Verification items for the finished model (mm, model axes). A direction names the side the tool comes from. Give positions to 0.01 mm unless a question says otherwise; leave off trailing zeros. Loops run counter-clockwise (first coordinate to the right, second up) from the corner with the lowest first, then second, coordinate; pieces in that order, holes last. Notation, with made-up numbers: M 63.5,-39 L 99.5,-39 A15 cw 99.5,-24 Z; hole C 45.25,62.5 d5. An arc over 180 degrees is marked long. Answer in a Markdown table with one row per item.
```python
from build123d import *

# Parameters (mm, degrees)
F0_W      = 15
F0_H      = 14.771302
F1_DEPTH  = 15
F2_R      = 4.5
F3_DEPTH  = 13.75
F4_R      = 4.5
F5_DEPTH  = 13.75
F6_R      = 4.5
F7_DEPTH  = 13.75
F8_R      = 1.575
F9_DEPTH  = 15.001
F10_R     = 1.575
F11_DEPTH = 14.772302
F12_R     = 1.575
F13_DEPTH = 15.001


with BuildPart() as f1:
    # F0 (on Front) → F1 (new body)
    with BuildSketch(Plane.XZ):
        Rectangle(F0_W, F0_H)
    extrude(amount=F1_DEPTH)

    # F2 (on face) → F3 (cut)
    with BuildSketch(Plane.XZ.offset(15)):
        Circle(F2_R)
    extrude(amount=-F3_DEPTH, mode=Mode.SUBTRACT)

    # F4 (on face) → F5 (cut)
    with BuildSketch(Plane.XY.offset(7.385651)):
        with Locations((0, -7.5)):
            Circle(F4_R)
    extrude(amount=-F5_DEPTH, mode=Mode.SUBTRACT)

    # F6 (on face) → F7 (cut)
    with BuildSketch(Plane(origin=(-7.5, 0, 0), x_dir=(0, -1, 0), z_dir=(-1, 0, 0))):
        with Locations((7.5, 0)):
            Circle(F6_R)
    extrude(amount=-F7_DEPTH, mode=Mode.SUBTRACT)

    # F8 (on face) → F9 (cut, through all)
    with BuildSketch(Plane(origin=(0, 0, 0), x_dir=(-1, 0, 0), z_dir=(0, 1, 0))):
        Circle(F8_R)
    extrude(amount=-F9_DEPTH, mode=Mode.SUBTRACT)

    # F10 (on face) → F11 (cut, through all)
    with BuildSketch(Plane(origin=(0, 0, -7.385651), x_dir=(1, 0, 0), z_dir=(0, 0, -1))):
        with Locations((0, 7.5)):
            Circle(F10_R)
    extrude(amount=-F11_DEPTH, mode=Mode.SUBTRACT)

    # F12 (on face) → F13 (cut, through all)
    with BuildSketch(Plane.YZ.offset(7.5)):
        with Locations((-7.5, 0)):
            Circle(F12_R)
    extrude(amount=-F13_DEPTH, mode=Mode.SUBTRACT)


solid = f1.part
```
Item 1: Sectioned sample at A-A (y = -7.5). Record the cut outline in (x, z) (3 decimals), and give its area (3 significant figures).
Reported:
| item | result |
|---|---|
| outline | M -7.5,-7.386 L -1.575,-7.386 L -1.575,-6.364 L -4.5,-6.364 L -4.5,-4.5 L -7.5,-4.5 Z; M -7.5,4.5 L -4.5,4.5 L -4.5,7.386 L -7.5,7.386 Z; M 1.575,-7.386 L 7.5,-7.386 L 7.5,-1.575 L 6.25,-1.575 L 6.25,-4.5 L 4.5,-4.5 L 4.5,-6.364 L 1.575,-6.364 Z; M 4.5,4.5 L 6.25,4.5 L 6.25,1.575 L 7.5,1.575 L 7.5,7.386 L 4.5,7.386 Z |
| area | 47.9 mm^2 |
Item 2: Go/stop test with a flat-tipped pin: pin 1 (5.5 mm diameter, centred on x = 0, y = -7.5, fed in from +Z). Record where the tip stops, or that it passes through.
Reported:
| item | result |
|---|---|
| pin 1 | stops at z = -6.36 |
Item 3: Sectioned sample at C-C (x = 4). Record the cut outline in (y, z).
Reported:
| item | result |
|---|---|
| outline | M -15,-7.39 L 0,-7.39 L 0,7.39 L -5.44,7.39 L -5.44,4 A4.5 cw -3.5,2.06 L -1.25,2.06 L -1.25,-2.06 L -3.5,-2.06 A4.5 cw -5.44,-4 L -5.44,-6.36 L -9.56,-6.36 L -9.56,-4 A4.5 cw -11.5,-2.06 L -15,-2.06 Z; M -15,2.06 L -11.5,2.06 A4.5 cw -9.56,4 L -9.56,7.39 L -15,7.39 Z |
Item 4: Tool access check on faces 4 (the cylindrical face through (-0.59, -3.04, 5.78)), 5 (the cylindrical face through (-3.32, -13.35, 3.04)), 6 (the cylindrical face through (5.04, -4.18, 3.04)). Record the directions out of +Z, -Z, +X, -X, +Y, -Y that give a thin tool (end or side, any length) a straight path to the whole face; none if there is none.
Reported:
| item | result |
|---|---|
| face 4 | +Z |
| face 5 | -Y |
| face 6 | -X |
Item 5: Scan lines: L1, parallel to Y at x = 5.5, z = 0; L2, parallel to Z at x = 6.8, y = -7.5 (3 decimals); L3, parallel to Y at x = 0, z = -7.2 (3 decimals). Record each from-to range of solid material in increasing order. Write a range as [from, to].
Reported:
| item | result |
|---|---|
| L1 | y = [-15, -12], [-3, 0] |
| L2 | z = [-7.386, -1.575], [1.575, 7.386] |
| L3 | y = [-15, -9.075], [-5.925, 0] |
Item 6: Sectioned sample at D-D (z = 5.5). Record the cut outline in (x, y), and give its area (3 significant figures).
Reported:
| item | result |
|---|---|
| outline | M -7.5,-15 L 7.5,-15 L 7.5,0 L -7.5,0 Z; hole C 0,-7.5 d9 |
| area | 161 mm^2 |
Item 7: Release check for a two-part mould opening along Z. For faces 1 (the flat face through (-2, -7, -7.386)), 2 (the flat face through (-3.4, -10.7, 7.386)), 3 (the cylindrical face through (-3.32, -2.46, 3.04)) record: released by +Z, released by -Z, zero draft, split by the parting line, or undercut.
Reported:
| item | result |
|---|---|
| face 1 | released by -Z |
| face 2 | released by +Z |
| face 3 | undercut |
Item 8: Sectioned sample at B-B (z = 0). Record the cut outline in (x, y) (3 decimals).
Reported:
| item | result |
|---|---|
| outline | M -7.5,-15 L -4.5,-15 L -4.5,-12 L -7.5,-12 Z; M -7.5,-3 L -4.5,-3 L -4.5,-1.25 L -1.575,-1.25 L -1.575,0 L -7.5,0 Z; M 1.575,-1.25 L 4.5,-1.25 L 4.5,-3 L 6.25,-3 L 6.25,-5.925 L 7.5,-5.925 L 7.5,0 L 1.575,0 Z; M 4.5,-15 L 7.5,-15 L 7.5,-9.075 L 6.25,-9.075 L 6.25,-12 L 4.5,-12 Z |
